The listing builds one solid part. Answer for the finished solid, in the listing's coordinates (mm). Coordinates: 2 decimals unless noted, no trailing zeros. Order: outer loops, then holes, each group sorted by start corner. A loop starts at its lowest first (then second) coordinate and runs counter-clockwise, first axis right, second up. Notation, with made-up numbers: (24.5, 71) -> (42.5, 71) arc R19 ccw to (42.5, 83) -> close; hole circle Ø6 at (16, -4.75). An arc over 180 degrees is marked (long way). Write each question's results on one line, items separated by ' | '. Start each with the question number.
(1) The part is cut by section C-C, the plane y = -11. Give the vertices of the cut face in (x, z).
(2) Straight lines are drawn through the part: L1, parallel to X at y = -49, z = 1.8; L2, parallel to Y at x = -1.5, z = 1.8; L3, parallel to X at y = -19, z = 1. For each, find the intervals that lie inside material, in ascending order.
(3) The part is cut by section A-A, the plane z = 0.55. Give the vertices of the cut face in (x, y), then the cut area to 3 significant figures.
(4) The part is cut by section B-B, the plane x = -11. Give the vertices of the cut face in (y, z), then the cut area to 3 significant figures.
```python
from build123d import *

# Parameters (mm, degrees)
RESSALTO_EXTRUS_O1_DEPTH = 3
FILETE1_R                = 5


with BuildPart() as part:
    # Esboço1 → Ressalto-extrusão1 (new body)
    with BuildSketch(Plane.XY):
        Polygon((0, 0), (24.9, 0), (39.140979909, -74.653831055), (-51.692763366, -74.653831055), align=None)
    extrude(amount=RESSALTO_EXTRUS_O1_DEPTH)

    # Filete1
    filete1_edges = [part.edges().sort_by_distance(p)[0] for p in [
        (24.9, 0, 1.5),
        (39.140979909, -74.653831055, 1.5),
    ]]
    fillet(filete1_edges, radius=FILETE1_R)


solid = part.part
```
Established:
1) outline: (-7.62, 0) -> (27, 0) -> (27, 3) -> (-7.62, 3) -> close
2) L1: x = -33.93 to 34.25 | L2: y = -74.65 to -2.17 | L3: x = -13.16 to 28.52
3) outline: (-51.69, -74.65) -> (33.1, -74.65) arc R5 ccw to (38.01, -68.72) -> (25.68, -4.06) arc R5 ccw to (20.76, 0) -> (0, 0) -> close | area: 4,310 mm^2
4) outline: (-74.65, 0) -> (-15.89, 0) -> (-15.89, 3) -> (-74.65, 3) -> close | area: 176 mm^2
